```python
from build123d import *

# Parameters (mm, degrees)
F0_R     = 2
F1_DEPTH = 2


with BuildPart() as f1:
    # F0 (on Front) → F1 (new body, symmetric)
    with BuildSketch(Plane.XZ):
        with BuildLine():
            ThreePointArc((2.8284271247, -2.8284271247), (3.69551813, -1.5307337295), (4, 0))
            ThreePointArc((4, 0), (3.69551813, 1.5307337295), (2.8284271247, 2.8284271247))
            ThreePointArc((2.8284271247, 2.8284271247), (1.5307337295, 3.69551813), (0, 4))
            ThreePointArc((0, 4), (-1.5307337295, 3.69551813), (-2.8284271247, 2.8284271247))
            ThreePointArc((-2.8284271247, 2.8284271247), (-3.69551813, 1.5307337295), (-4, 0))
            ThreePointArc((-4, 0), (-3.69551813, -1.5307337295), (-2.8284271247, -2.8284271247))
            ThreePointArc((-2.8284271247, -2.8284271247), (-1.5307337295, -3.69551813), (0, -4))
            ThreePointArc((0, -4), (1.5307337295, -3.69551813), (2.8284271247, -2.8284271247))
        make_face()
        Circle(F0_R, mode=Mode.SUBTRACT)
        with BuildLine():
            Line((5.8637033052, -2.4288254347), (4, 0))
            ThreePointArc((4, 0), (3.69551813, -1.5307337295), (2.8284271247, -2.8284271247))
            Line((2.8284271247, -2.8284271247), (5.8637033052, -2.4288254347))
        make_face()
        with BuildLine():
            ThreePointArc((2.8284271247, 2.8284271247), (3.69551813, 1.5307337295), (4, 0))
            Line((4, 0), (5.8637033052, 2.4288254347))
            Line((5.8637033052, 2.4288254347), (2.8284271247, 2.8284271247))
        make_face()
        with BuildLine():
            ThreePointArc((0, 4), (1.5307337295, 3.69551813), (2.8284271247, 2.8284271247))
            Line((2.8284271247, 2.8284271247), (2.4288254347, 5.8637033052))
            Line((2.4288254347, 5.8637033052), (0, 4))
        make_face()
        with BuildLine():
            Line((2.4288254347, -5.8637033052), (2.8284271247, -2.8284271247))
            ThreePointArc((2.8284271247, -2.8284271247), (1.5307337295, -3.69551813), (0, -4))
            Line((0, -4), (2.4288254347, -5.8637033052))
        make_face()
        with BuildLine():
            ThreePointArc((-2.8284271247, 2.8284271247), (-1.5307337295, 3.69551813), (0, 4))
            Line((0, 4), (-2.4288254347, 5.8637033052))
            Line((-2.4288254347, 5.8637033052), (-2.8284271247, 2.8284271247))
        make_face()
        with BuildLine():
            Line((-2.4288254347, -5.8637033052), (0, -4))
            ThreePointArc((0, -4), (-1.5307337295, -3.69551813), (-2.8284271247, -2.8284271247))
            Line((-2.8284271247, -2.8284271247), (-2.4288254347, -5.8637033052))
        make_face()
        with BuildLine():
            ThreePointArc((-4, 0), (-3.69551813, 1.5307337295), (-2.8284271247, 2.8284271247))
            Line((-2.8284271247, 2.8284271247), (-5.8637033052, 2.4288254347))
            Line((-5.8637033052, 2.4288254347), (-4, 0))
        make_face()
        with BuildLine():
            Line((-5.8637033052, -2.4288254347), (-2.8284271247, -2.8284271247))
            ThreePointArc((-2.8284271247, -2.8284271247), (-3.69551813, -1.5307337295), (-4, 0))
            Line((-4, 0), (-5.8637033052, -2.4288254347))
        make_face()
    extrude(amount=F1_DEPTH, both=True)


solid = f1.part
```
Can you work these out from the model? Positions are in its coordinate system, mm. A direction names the side the tool comes from. Coordinates: 2 decimals unless noted, no trailing zeros. Loops run counter-clockwise (first coordinate to the right, second up) from the corner with the lowest first, then second, coordinate; pieces in that order, holes last. Notation, with made-up numbers: (-9, 43) -> (7, 43) arc R16 cw to (7, 74) -> close; hole circle Ø1 at (43, 34). An arc over 180 degrees is marked (long way). Put each result on its own line as item: value. Start each with the question number.
Q1. I want a section at C-C (x = -4.5). Write out the boundary of the cut face in (y, z), plus the area to 3 significant figures.
Q2. I want a section at D-D (z = -3.75). Write out the boundary of the cut face in (x, y).
Q3. Thinking about a two-plate mould opening in X: for faces 5 (the face through (0, -2, -3)), 6 (the face through (1.231, -0.028, 4.945)), 7 (the face through (2.626, -0.028, -4.367)), which applies, pulls with the +X half, pulls with the -X half, needs draft (parallel to the pull), parting line crosses it, or undercut?
Q4. I want a section at B-B (z = -1.5). Write out the boundary of the cut face in (x, y), plus the area to 3 significant figures.
Q5. I want a section at A-A (y = -1.3). Write out the boundary of the cut face in (x, z).
Q6. If I drill on line 1 (Z direction, x = -1.75, y = 0.4); line 2 (Z direction, x = -0.75, y = -1.3); line 3 (X direction, y = -0.2, z = -3.5), over which ranges is the centre line in solid material (lowest first)? Write a range as [from, to].
Q7. For faces 1 (the face through (-1.231, -0.028, -4.945)), 2 (the face through (4.92, -0.03, 1.2)), 3 (the face through (-4.92, -0.03, -1.2)), 4 (the face through (-1.2, -0.03, 4.92)), which set-ups out of +Z, -Z, +X, -X, +Y, -Y let a thin tool reach every point of the face, with its end or its side?
Taken from the geometry:
1. outline: (-2, -2.61) -> (2, -2.61) -> (2, -0.65) -> (-2, -0.65) -> close; (-2, 0.65) -> (2, 0.65) -> (2, 2.61) -> (-2, 2.61) -> close
1. area: 15.7 mm2
2. outline: (-2.71, -2) -> (2.71, -2) -> (2.71, 2) -> (-2.71, 2) -> close
3. face 5: needs draft
3. face 6: undercut
3. face 7: pulls with the +X half
4. outline: (-5.15, -2) -> (-1.32, -2) -> (-1.32, 2) -> (-5.15, 2) -> close; (1.32, -2) -> (5.15, -2) -> (5.15, 2) -> (1.32, 2) -> close
4. area: 30.6 mm2
5. outline: (-5.86, -2.43) -> (-2.83, -2.83) -> (-2.43, -5.86) -> (0, -4) -> (2.43, -5.86) -> (2.83, -2.83) -> (5.86, -2.43) -> (4, 0) -> (5.86, 2.43) -> (2.83, 2.83) -> (2.43, 5.86) -> (0, 4) -> (-2.43, 5.86) -> (-2.83, 2.83) -> (-5.86, 2.43) -> (-4, 0) -> close; hole circle Ø4 at (0, 0)
6. line 1: z = [-5.34, -0.97], [0.97, 5.34]
6. line 2: z = [-4.58, -1.85], [1.85, 4.58]
6. line 3: x = [-2.74, 2.74]
7. face 1: -Z, +Y, -Y
7. face 2: +X, +Y, -Y
7. face 3: -X, +Y, -Y
7. face 4: +Z, +Y, -Y
